```python
from build123d import *

# Parameters (mm, degrees)
F0_W     = 14
F0_H     = 69
F0_R     = 4
F1_DEPTH = 14
F2_R     = 3.2
F3_DEPTH = 14.001
F4_DEPTH = 6
F5_R     = 5


with BuildPart() as f1:
    # F0 (on Top) → F1 (new body)
    with BuildSketch(Plane.XY):
        with Locations((7, 34.5)):
            Rectangle(F0_W, F0_H)
        with Locations((7, 10)):
            Circle(F0_R, mode=Mode.SUBTRACT)
        with Locations((7, 28)):
            Circle(F0_R, mode=Mode.SUBTRACT)
        with Locations((7, 46)):
            Circle(F0_R, mode=Mode.SUBTRACT)
    extrude(amount=F1_DEPTH)

    # F2 (on face) → F3 (cut, through all)
    with BuildSketch(Plane(origin=(0, 0, 0), x_dir=(0, -1, 0), z_dir=(-1, 0, 0))):
        with Locations((-61, 7)):
            Circle(F2_R)
    extrude(amount=-F3_DEPTH, mode=Mode.SUBTRACT)

    # F2 (on face) → F4 (cut)
    with BuildSketch(Plane(origin=(0, 0, 0), x_dir=(0, -1, 0), z_dir=(-1, 0, 0))):
        Polygon((-63.944486, 1.9), (-58.055514, 1.9), (-55.111027, 7), (-58.055514, 12.1), (-63.944486, 12.1), (-66.888973, 7), align=None)
        with Locations((-61, 7)):
            Circle(F2_R, mode=Mode.SUBTRACT)
    extrude(amount=-F4_DEPTH, mode=Mode.SUBTRACT)

    # F5
    f5_edges = [f1.edges().sort_by_distance(p)[0] for p in [
        (7, 69, 14),
        (7, 69, 0),
    ]]
    fillet(f5_edges, radius=F5_R)


solid = f1.part
```
Geometry check sheet. Reference: the model listing, model coordinates, mm. A direction names the side the tool comes from. Give positions to 0.01 mm unless a question says otherwise; leave off trailing zeros. Order: outer loops, then holes, each group sorted by start corner. A loop starts at its lowest first (then second) coordinate and runs counter-clockwise, first axis right, second up. Notation, with made-up numbers: (73.25, 29) - (123.25, 29) arc R12 ccw to (123.25, 50) - close; hole circle Ø6 at (27, 42.5). An arc over 180 degrees is marked (long way). Write item = value, one per line. Start each with the question number.
1) Gauge pin test, flat ends, axial feed: pin 1 Ø7 at (x, y) = (7, 46) entering from -Z; pin 2 Ø5 at (x, y) = (10, 12.5) entering from +Z; pin 3 Ø1.5 at (x, z) = (4, 10) entering from +Y. Record the tip position at first contact, or that the pin passes through.
2) Draft check along Y on faces 1 (the flat face through (0, 34, 7)), 2 (the cylindrical face through (6.479, 31.966, 6.902)), 3 (the flat face through (7, 0, 7)). Enter one of: released by +Y, released by -Y, zero draft, split by the parting line, or undercut.
3) Section check C-C (z = 13). Enter the section's corners in (x, y).
4) Section check D-D (z = 5.75). Enter the section's corners in (x, y).
5) Section check A-A (y = 28). Enter the section's corners in (x, z), then the cut area to 3 significant figures.
6) Access from +Z, -Z, +X, -X, +Y, -Y to the whole of each face (thin tool, end or side, straight path). Record for faces 4 (the flat face through (2.96, 56.56, 9.51)), 5 (the cylindrical face through (9.9, 64.2, 7.1)).
7) Scan lines: L1, parallel to Y at x = 9.5, z = 3.25; L2, parallel to Y at x = 5.5, z = 4.5; L3, parallel to Y at x = 5.25, z = 7.25. Record each from-to range of solid material in increasing order.
8) Section check B-B (x = 7). Enter the section's corners in (y, z), then the cut area to 3 significant figures.
Geometry check:
q1.pin_1 = through
q1.pin_2 = 14
q1.pin_3 = 68.99
q2.face_1 = zero draft
q2.face_2 = undercut
q2.face_3 = released by -Y
q3.outline = (0, 0) - (14, 0) - (14, 67) - (0, 67) - close; hole circle Ø8 at (7, 10); hole circle Ø8 at (7, 28); hole circle Ø8 at (7, 46)
q4.outline = (0, 0) - (14, 0) - (14, 58.05) - (6, 58.05) - (6, 55.83) - (0, 55.83) - close; (0, 66.17) - (6, 66.17) - (6, 63.95) - (14, 63.95) - (14, 69) - (0, 69) - close; hole circle Ø8 at (7, 10); hole circle Ø8 at (7, 28); hole circle Ø8 at (7, 46)
q5.outline = (0, 0) - (3, 0) - (3, 14) - (0, 14) - close; (11, 0) - (14, 0) - (14, 14) - (11, 14) - close
q5.area = 84.0 mm2
q6.face_4 = -X
q6.face_5 = +X, -X
q7.L1 = 0 to 6.88, 13.12 to 24.88, 31.12 to 42.88, 49.12 to 68.68
q7.L2 = 0 to 6.29, 13.71 to 24.29, 31.71 to 42.29, 49.71 to 56.55, 65.45 to 68.97
q7.L3 = 0 to 6.4, 13.6 to 24.4, 31.6 to 42.4, 49.6 to 55.26, 66.74 to 69
q8.outline = (0, 0) - (6, 0) - (6, 14) - (0, 14) - close; (14, 0) - (24, 0) - (24, 14) - (14, 14) - close; (32, 0) - (42, 0) - (42, 14) - (32, 14) - close; (50, 0) - (64, 0) arc R5 ccw to (69, 5) - (69, 9) arc R5 ccw to (64, 14) - (50, 14) - close; hole circle Ø6.4 at (61, 7)
q8.area = 587 mm2
